Geometry: final body of the model. Coordinates: model frame, mm. A direction names the side the tool comes from. Give positions to 0.01 mm unless a question says otherwise; leave off trailing zeros. Order: outer loops, then holes, each group sorted by start corner. A loop starts at its lowest first (then second) coordinate and runs counter-clockwise, first axis right, second up. Notation, with made-up numbers: (68.5, -33.5) -> (126.5, -33.5) arc R15 ccw to (126.5, -18.5) -> close; hole circle Ø6 at (6.5, -30.5). An arc over 180 degrees is marked (long way). One line per question, with ' | ' between items. Start each with the question number.
(1) Section B-B (z = -3.8). Return loops of the section in (x, y).
(2) Set-up query: faces 5 (the face through (-145.102, 44.114, 0.406)), 6 (the face through (-76, 1.6, -2)), 7 (the face through (-111.125, 61.206, -4.251)). Return all of +Z, -Z, +X, -X, +Y, -Y with unobstructed straight access to the full face (end or side cutting, diameter ignored); none if empty.
(3) Section A-A (y = 43.1). Return loops of the section in (x, z).
(4) Ray query, L1, parallel to X at y = 61.4, z = -3.8; L2, parallel to Y at x = -24.5, z = -4.5; L3, parallel to Y at x = -112.5, z = -3.75. Return the intervals inside material, ascending.
(5) Section D-D (y = 18.1). Return loops of the section in (x, z).
(6) Section C-C (x = -25.5). Return loops of the section in (y, z), then the cut area to 3 significant figures.
(7) First-contact query: pin 1 Ø5 at (x, y) = (-144, 18.1) entering from +Z; pin 2 Ø2 at (x, y) = (-30.5, 29.5) entering from -Z; pin 3 Ø2.5 at (x, y) = (-6.11, 43.1) entering from -Z; pin 4 Ø1.8 at (x, z) = (-112.56, -3.8) entering from +Y. Flat tips, straight axial feed; report the tip coordinate or a pass-through.
(8) Mould query, pull axis Y, two halves, no side actions, for faces 1 (the face through (-74, 61.6, -5)), 2 (the face through (0, 31.3, 0.2)), 3 (the face through (-7.22, 19.114, 0.406)), 4 (the face through (-76, 0.8, -1)). Classes: +Y half, -Y half, draft (parallel to the pull), parting line (faces both ways), or undercut.
Autodesk Inventor part; units mm, degrees
ref_plane "YZ Plane" through (0, 0, 0) normal (1, 0, 0) x (0, 1, 0)
ref_plane "XZ Plane" through (0, 0, 0) normal (0, 1, 0) x (-1, 0, 0)
ref_plane "XY Plane" through (0, 0, 0) normal (0, 0, 1) x (1, 0, 0)
ref_plane "Płaszczyzna konstrukcyjna1" through (0, 0, 0) normal (0, 0, 1) x (1, 0, 0)
sketch "Szkic2" plane through (0, 0, 0) normal (0, 0, 1) x (1, 0, 0)
  line L0 (0, 0.8) -> (-150.1111, 0.8)
  line L1 (-150.1111, 0) -> (-150.1111, 0.8)
  line L2 (0, 0) -> (-150.1111, 0)
  line L3 (0, 0) -> (0, 0.8)
  line L4 (-150.1111, 0) -> (0, 0)
  line L5 (0, 0) -> (0, 60)
  line L6 (0, 60) -> (-150.1111, 60)
  line L7 (-150.1111, 60) -> (-150.1111, 0)
  dimension "d0" = 60
extrude "Płyta1" add sketch "Szkic2" along normal blind 0.8 contours L0 L7 L6 L5
sketch "Szkic3" plane through (-150.1111, 1.6, 0.8) normal (0, -1, 0) x (1, 0, 0)
  line L0 (150.1111, 0) -> (0, 0)
  line L1 (0, 0) -> (0, -10)
  line L2 (0, -10) -> (150.1111, -10)
  line L3 (150.1111, -10) -> (150.1111, 0)
edge flange "Kołnierz1" height 10 angle 90 thickness 0.8 bend radius 0.8 thickness toward (0, -1, 0) relief straight relief width 0.8 relief depth 0.4 edges at (-75.0555, 0.8, 0) wall of the first edge with corners at (0, 1.6, 0.8) (-150.1111, 1.6, 0.8) (-150.1111, 1.6, -9.2) (0, 1.6, -9.2)
bend "Gięcie1"
corner "Narożnik1"
sketch "Szkic4" plane through (0, 60.8, -0.8) normal (0, 1, 0) x (-1, 0, 0)
  line L0 (150.1111, 0) -> (0, 0)
  line L1 (0, 0) -> (0, -8.4)
  line L2 (0, -8.4) -> (150.1111, -8.4)
  line L3 (150.1111, -8.4) -> (150.1111, 0)
edge flange "Kołnierz2" height 10 angle 90 thickness 0.8 bend radius 0.8 thickness toward (0, 1, 0) relief straight relief width 0.8 relief depth 0.4 edges at (-75.0555, 60, 0) wall of the first edge with corners at (-150.1111, 60.8, -0.8) (0, 60.8, -0.8) (0, 60.8, -9.2) (-150.1111, 60.8, -9.2)
bend "Gięcie2"
corner "Narożnik2"
sketch "Szkic5" plane through (-150.1111, 0.8, -9.2) normal (0, -1, 0) x (1, 0, 0)
  line L0 (150.1111, 0) -> (0, 0)
  line L1 (0, 0) -> (150.1111, 0) construction
  line L2 (75.0555, 0) -> (75.0555, 31.3517) construction
  line L3 (52.5555, 0) -> (97.5555, 0)
  line L4 (97.5555, 0) -> (97.5555, 7)
  line L5 (97.5555, 7) -> (52.5555, 7)
  line L6 (52.5555, 7) -> (52.5555, 0)
  point P0 (150.1111, 9.2)
  dimension "d22" = 7
  dimension "d23" = 45
extrude "Wytnij1" cut sketch "Szkic5" against normal blind 0.8
sketch "Szkic6" plane through (-150.1111, 61.6, -9.2) normal (0, 1, 0) x (1, 0, 0)
  circle A0 centre (37.5555, -5.4) radius 1.5
  circle A1 centre (112.5555, -5.4) radius 1.5
  point P0 (150.1111, -9.2)
extrude "Wytnij2" cut sketch "Szkic6" against normal blind 0.8
sketch "Szkic7" plane through (0, 0, 0.8) normal (0, 0, 1) x (1, 0, 0)
  circle A0 centre (-143.9967, 43.1) radius 1.5
  circle A1 centre (-143.9967, 18.1) radius 1.5
  circle A2 centre (-6.1144, 18.1) radius 1.5
  circle A3 centre (-6.1144, 43.1) radius 1.5
  point P0 (0, 0)
extrude "Wytnij3" cut sketch "Szkic7" against normal blind 0.8
sketch "Szkic8" plane through (0, 0, 0.8) normal (0, 0, 1) x (1, 0, 0)
  circle A0 centre (-75.0555, 20.8) radius 7.5
  point P0 (0, 0)
  dimension "d30" = 15
extrude "Wytnij4" cut sketch "Szkic8" against normal blind 0.8
equation "\"d24\" = Grubość"
equation "\"d26\" = Grubość"
equation "\"d28\" = Grubość"
equation "\"d31\" = Grubość"
equation "\"d2\" = SzerokośćGięciaPodcięcia"
equation "\"d3\" = GłębokośćGięciaPodcięcia"
equation "\"d4\" = MinimalnaPozostałość"
equation "\"d5\" = PromieńGięcia"
equation "\"d8\" = PromieńGięcia"
equation "\"d9\" = RozmiarPodcięciaNarożnika"
equation "\"d10\" = Wielk_odstępu"
equation "\"d11\" = Rozmiar_promienia_Jacobiego"
equation "\"d12\" = SzerokośćGięciaPodcięcia"
equation "\"d13\" = GłębokośćGięciaPodcięcia"
equation "\"d14\" = MinimalnaPozostałość"
equation "\"d15\" = PromieńGięcia"
equation "\"d18\" = PromieńGięcia"
equation "\"d19\" = RozmiarPodcięciaNarożnika"
equation "\"d20\" = Wielk_odstępu"
equation "\"d21\" = Rozmiar_promienia_Jacobiego"
equation "\"PromieńGięcia\" = Grubość"
equation "\"SzerokośćGięciaPodcięcia\" = Grubość"
equation "\"GłębokośćGięciaPodcięcia\" = 0.5 * Grubość"
equation "\"RozmiarPodcięciaNarożnika\" = 4 * Grubość"
equation "\"MinimalnaPozostałość\" = 2 * Grubość"
equation "\"PromieńPrzejścia\" = PromieńGięcia"
equation "\"Rozmiar_promienia_Jacobiego\" = Grubość"
equation "\"Wielk_odstępu\" = Grubość"
equation "\"d1\" = PromieńGięcia"
properties part number "base_side_constr"
Response:
1) outline: (-150.11, 0.8) -> (-97.56, 0.8) -> (-97.56, 1.6) -> (-150.11, 1.6) -> close; (-150.11, 60.8) -> (-114.06, 60.8) -> (-114.06, 61.6) -> (-150.11, 61.6) -> close; (-111.06, 60.8) -> (-39.06, 60.8) -> (-39.06, 61.6) -> (-111.06, 61.6) -> close; (-52.56, 0.8) -> (0, 0.8) -> (0, 1.6) -> (-52.56, 1.6) -> close; (-36.06, 60.8) -> (0, 60.8) -> (0, 61.6) -> (-36.06, 61.6) -> close
2) face 5: +Z, -Z | face 6: -Z, +X, -X | face 7: +Y
3) outline: (-150.11, 0) -> (-145.5, 0) -> (-145.5, 0.8) -> (-150.11, 0.8) -> close; (-142.5, 0) -> (-7.61, 0) -> (-7.61, 0.8) -> (-142.5, 0.8) -> close; (-4.61, 0) -> (0, 0) -> (0, 0.8) -> (-4.61, 0.8) -> close
4) L1: x = -150.11 to -114.06, -111.06 to -39.06, -36.06 to 0 | L2: y = 0.8 to 1.6, 60.8 to 61.6 | L3: y = 0.8 to 1.6
5) outline: (-150.11, 0) -> (-145.5, 0) -> (-145.5, 0.8) -> (-150.11, 0.8) -> close; (-142.5, 0) -> (-82.05, 0) -> (-82.05, 0.8) -> (-142.5, 0.8) -> close; (-68.06, 0) -> (-7.61, 0) -> (-7.61, 0.8) -> (-68.06, 0.8) -> close; (-4.61, 0) -> (0, 0) -> (0, 0.8) -> (-4.61, 0.8) -> close
6) outline: (0.8, -9.2) -> (1.6, -9.2) -> (1.6, -0.8) arc R0.8 cw to (2.4, 0) -> (60, 0) arc R0.8 cw to (60.8, -0.8) -> (60.8, -9.2) -> (61.6, -9.2) -> (61.6, -0.8) arc R1.6 ccw to (60, 0.8) -> (2.4, 0.8) arc R1.6 ccw to (0.8, -0.8) -> close | area: 62.5 mm^2
7) pin 1: stops at z = 0.8 | pin 2: stops at z = 0 | pin 3: passes through | pin 4: stops at y = 1.6
8) face 1: +Y half | face 2: draft | face 3: undercut | face 4: -Y half
